from build123d import *

# Parameters (mm, degrees)
F0_R     = 2.5
F1_DEPTH = 25
F2_R     = 7
F3_DEPTH = 12.5
F5_DEPTH = 25
F6_R     = 2.75
F7_DEPTH = 25
F8_SIZE  = 2
F9_SIZE  = 1.5


with BuildPart() as f1:
    # F0 (on Right) → F1 (new body)
    with BuildSketch(Plane.YZ):
        with BuildLine():
            Line((34.771998, -1.392547), (13.660271, -0.839717))
            Line((13.660271, -0.839717), (10.68098, -6))
            Line((10.68098, -6), (7.072541, -12.25))
            Line((7.072541, -12.25), (-7.072541, -12.25))
            Line((-7.072541, -12.25), (-10.68098, -6))
            Line((-10.68098, -6), (-14.145082, 0))
            ThreePointArc((-14.145082, 0), (-18.998978, -5.88952), (-25.70723, -2.25))
            Line((-25.70723, -2.25), (-50.145082, -2.25))
            Line((-50.145082, -2.25), (-50.145082, -14.25))
            Line((-50.145082, -14.25), (-15.155445, -14.25))
            Line((-15.155445, -14.25), (-12.846043, -18.25))
            ThreePointArc((-12.846043, -18.25), (-11.381942, -19.714102), (-9.381942, -20.25))
            Line((-9.381942, -20.25), (9.381942, -20.25))
            ThreePointArc((9.381942, -20.25), (11.381942, -19.714102), (12.846043, -18.25))
            Line((12.846043, -18.25), (15.299782, -14))
            ThreePointArc((15.299782, -14), (16.809399, -12.510016), (18.868592, -12.001371))
            Line((18.868592, -12.001371), (30.48486, -12.305553))
            ThreePointArc((30.48486, -12.305553), (33.342986, -11.208422), (34.588197, -8.411632))
            Line((34.588197, -8.411632), (34.771998, -1.392547))
        make_face()
        Polygon((25.287627, -9.3256), (23.83504, -9.287563), (23.422342, -7.894316), (24.619867, -7.07128), (25.772677, -7.955862), align=None, mode=Mode.SUBTRACT)
        with BuildLine():
            ThreePointArc((-25.70723, -2.25), (-18.998978, -5.88952), (-14.145082, 0))
            ThreePointArc((-14.145082, 0), (-21.291185, 5.88952), (-25.70723, -2.25))
        make_face()
        with Locations((-20.145082, 0)):
            Circle(F0_R, mode=Mode.SUBTRACT)
    extrude(amount=F1_DEPTH)

    # F2 (on face) → F3 (cut)
    with BuildSketch(Plane.YZ.offset(25)):
        with Locations((-20.145082, 0)):
            Circle(F2_R)
    extrude(amount=-F3_DEPTH, mode=Mode.SUBTRACT)

    # F4 (on face) → F5 (cut)
    with BuildSketch(Plane(origin=(0, -0.301122, -11.499394), x_dir=(1, 0, 0), z_dir=(0, -0.026177, -0.999657))):
        with BuildLine():
            Line((9.5, -22.176285), (9.5, -27.796535))
            ThreePointArc((9.5, -27.796535), (12.5, -30.796535), (15.5, -27.796535))
            Line((15.5, -27.796535), (15.5, -22.176285))
            ThreePointArc((15.5, -22.176285), (12.5, -19.176285), (9.5, -22.176285))
        make_face()
    extrude(amount=-F5_DEPTH, mode=Mode.SUBTRACT)

    # F6 (on face) → F7 (cut)
    with BuildSketch(Plane.XY.offset(-2.25)):
        with Locations((12.5, -40.145082)):
            Circle(F6_R)
        with BuildLine():
            ThreePointArc((19.571068, -47.216149), (12.5, -50.145082), (5.428932, -47.216149))
            Line((5.428932, -47.216149), (-9.84301, -31.944207))
            Line((-9.84301, -31.944207), (-9.84301, -58.411797))
            Line((-9.84301, -58.411797), (34.84301, -58.411797))
            Line((34.84301, -58.411797), (34.84301, -31.944207))
            Line((34.84301, -31.944207), (19.571068, -47.216149))
        make_face()
    extrude(amount=-F7_DEPTH, mode=Mode.SUBTRACT)

    # F8
    f8_edges = [f1.edges().sort_by_distance(p)[0] for p in [
        (0, 24.216134, -1.116132),
        (0, 10.366406, -6.544858),
        (0, 0, -12.25),
        (0, -10.608811, -6.125),
        (0, -21.291185, 5.88952),
        (0, -14.000744, -16.25),
        (12.5, 34.771998, -1.392547),
        (25, 24.216134, -1.116132),
        (25, 10.366406, -6.544858),
        (25, 0, -12.25),
        (25, -10.186207, -6.856971),
        (25, -14.000744, -16.25),
        (25, -11.381942, -19.714102),
        (25, 0, -20.25),
        (25, 11.381942, -19.714102),
        (25, 14.072913, -16.125),
        (25, 24.676726, -12.153462),
        (25, 16.809399, -12.510016),
        (25, 33.342986, -11.208422),
        (25, 34.680097, -4.902089),
        (0, -11.381942, -19.714102),
        (0, 0, -20.25),
        (0, 11.381942, -19.714102),
        (0, 14.072913, -16.125),
        (0, 16.809399, -12.510016),
        (0, 24.676726, -12.153462),
        (0, 33.342986, -11.208422),
        (0, 34.680097, -4.902089),
    ]]
    chamfer(f8_edges, length=F8_SIZE)

    # F9
    f9_edges = [f1.edges().sort_by_distance(p)[0] for p in [
        (25, -28.471331, -14.25),
        (25, -34.280418, -2.25),
        (0, -33.747224, -2.25),
        (0, -28.471331, -14.25),
    ]]
    chamfer(f9_edges, length=F9_SIZE)


solid = f1.part
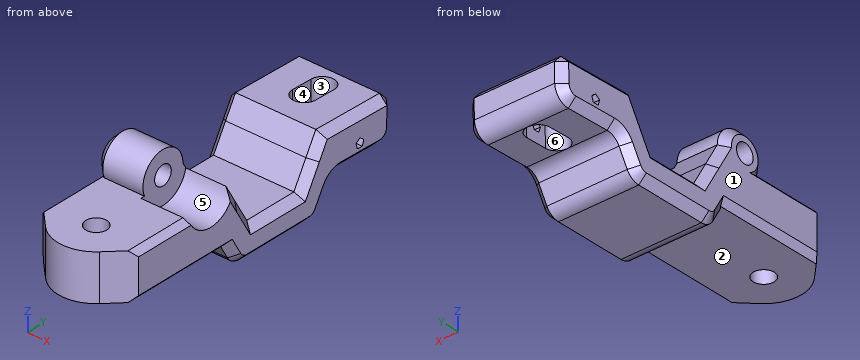
CAD build for the part. Positions are in the model's coordinates, mm. Face numbers are marked on the shaded views. A direction names the side the tool comes from. Round coordinates to 2 decimals unless told otherwise and drop trailing zeros. Loops run counter-clockwise (first coordinate to the right, second up) from the corner with the lowest first, then second, coordinate; pieces in that order, holes last.
(1) Which spindle directions (+Z, -Z, +X, -X, +Y, -Y) get a long thin tool onto all of the face, cutting with end or side? Do the marked faces 4, 5 and 6. Say none if no direction does.
(2) Cut at C-C (x = 18.75). Give the cut face in (y, z).
(3) Drop flat-ended pins along their axis: pin 1 (4 mm diameter, centred on x = 15, y = 2, fed in from +Z); pin 2 (12 mm diameter, centred on x = 14, y = 20, fed in from +Z); pin 3 (6.5 mm diameter, centred on y = -17.5, z = 0.5, fed in from +X). Give the stop position or say it passes through.
(4) Two-plate mould, pull along X, no slides. Class the marked faces 1, 2 and 3: +X half, -X half, draft (parallel to the pull), parting line (faces both ways), or undercut.
(5) Cut at A-A (y = -4.5). Give the cut face in (x, z).
(6) Cut at D-D (x = 22.25). Give the cut face in (y, z), plus the area to 3 significant figures.
(7) Cut at B-B (x = 6.25). Give the cut face in (y, z), plus the area to 3 significant figures.
(8) Wall check: line 1 along Y through (x, z) = (12.5, -11); line 2 along Z through (x, y) = (13.5, 0). Give the ranges that are in metal, low to high.
Findings below:
1. face 4: +Z, -Z
1. face 5: +Z, +X
1. face 6: -Z
2. outline: (-47.95, -14.25) - (-15.16, -14.25) - (-12.85, -18.25) arc R4 ccw to (-9.38, -20.25) - (9.38, -20.25) arc R4 ccw to (12.85, -18.25) - (15.3, -14) arc R4 cw to (18.87, -12) - (30.48, -12.31) arc R4 ccw to (34.59, -8.41) - (34.72, -3.39) - (32.77, -1.34) - (13.66, -0.84) - (7.07, -12.25) - (-7.07, -12.25) - (-13.3, -1.46) arc R7 cw to (-26.77, -2.25) - (-47.95, -2.25) - close; hole (23.42, -7.89) - (23.84, -9.29) - (25.29, -9.33) - (25.77, -7.96) - (24.62, -7.07) - close
3. pin 1: stops at z = -12.25
3. pin 2: stops at z = -0.85
3. pin 3: stops at x = 12.5
4. face 1: -X half
4. face 2: draft
4. face 3: undercut
5. outline: (0, -18.25) - (2, -20.25) - (23, -20.25) - (25, -18.25) - (25, -14.25) - (23, -12.25) - (2, -12.25) - (0, -14.25) - close
6. outline: (-44.54, -14.25) - (-15.16, -14.25) - (-12.85, -18.25) arc R4 ccw to (-9.38, -20.25) - (9.38, -20.25) arc R4 ccw to (12.85, -18.25) - (15.3, -14) arc R4 cw to (18.87, -12) - (30.48, -12.31) arc R4 ccw to (34.59, -8.41) - (34.72, -3.39) - (32.77, -1.34) - (13.66, -0.84) - (7.07, -12.25) - (-7.07, -12.25) - (-13.3, -1.46) arc R7 cw to (-26.77, -2.25) - (-44.54, -2.25) - close; hole (23.42, -7.89) - (23.84, -9.29) - (25.29, -9.33) - (25.77, -7.96) - (24.62, -7.07) - close
6. area: 841 mm2
7. outline: (-47.95, -14.25) - (-15.16, -14.25) - (-12.85, -18.25) arc R4 ccw to (-9.38, -20.25) - (9.38, -20.25) arc R4 ccw to (12.85, -18.25) - (15.3, -14) arc R4 cw to (18.87, -12) - (30.48, -12.31) arc R4 ccw to (34.59, -8.41) - (34.72, -3.39) - (32.77, -1.34) - (13.66, -0.84) - (7.07, -12.25) - (-7.07, -12.25) - (-14.15, 0) arc R6 ccw (long way) to (-25.71, -2.25) - (-47.95, -2.25) - close; hole circle Ø5 at (-20.15, 0); hole (23.42, -7.89) - (23.84, -9.29) - (25.29, -9.33) - (25.77, -7.96) - (24.62, -7.07) - close
7. area: 993 mm2
8. line 1: y = -50.15 to -42.9, -37.4 to -7.79, 7.79 to 18.89, 30.52 to 33.55
8. line 2: z = -20.25 to -12.25
